CAD build for the part. Positions are in the model's coordinates, mm. A direction names the side the tool comes from. Give positions to 0.01 mm unless a question says otherwise; leave off trailing zeros. Loops run counter-clockwise (first coordinate to the right, second up) from the corner with the lowest first, then second, coordinate; pieces in that order, holes last.
```python
from build123d import *

# Parameters (mm, degrees)
M3_THREAD_ENVELOPE_SELECT_HARDWARE_START = 40
SKETCH1_R                                = 1.5
M3_THREAD_ENVELOPE_SELECT_HARDWARE_DEPTH = 7.5
THUMB_HEAD_START                         = 47.5
SKETCH2_R                                = 4
THUMB_HEAD_DEPTH                         = 4
DRIVER_SLOT_START                        = 50
SKETCH3_W                                = 1.2
SKETCH3_H                                = 10
DRIVER_SLOT_DEPTH                        = 3


with BuildPart() as part:
    # Sketch1 → M3_thread_envelope_select_hardware (new body)
    with BuildSketch(Plane.XY.offset(M3_THREAD_ENVELOPE_SELECT_HARDWARE_START)):
        with Locations((-20, 0)):
            Circle(SKETCH1_R)
    extrude(amount=M3_THREAD_ENVELOPE_SELECT_HARDWARE_DEPTH)

    # Sketch2 → Thumb_head (add)
    with BuildSketch(Plane.XY.offset(THUMB_HEAD_START)):
        with Locations((-20, 0)):
            Circle(SKETCH2_R)
    extrude(amount=THUMB_HEAD_DEPTH)

    # Sketch3 → Driver_slot (cut)
    with BuildSketch(Plane.XY.offset(DRIVER_SLOT_START)):
        with Locations((-20, 0)):
            Rectangle(SKETCH3_W, SKETCH3_H)
    extrude(amount=DRIVER_SLOT_DEPTH, mode=Mode.SUBTRACT)


solid = part.part
```
1. Probe line 1 along Z through (x, y) = (-19.5, 3.25); line 2 along Z through (x, y) = (-22.75, -0.25); line 3 along Y through (x, z) = (-20, 44.5). List the from-to ranges inside material, lowest first.
Responses:
line 1: z = 47.5 to 50
line 2: z = 47.5 to 51.5
line 3: y = -1.5 to 1.5
2. Saw through at D-D, the plane z = 49. List the corners of the cut face in (x, y), and give its area (3 significant figures).
Responses:
outline: circle Ø8 at (-20, 0)
area: 50.3 mm2
3. Pull direction X, two halves, no side cores. Call faces 4 (the face through (-20.6, 0, 51)), 5 (the face through (-22, 0, 51.5)), 6 (the face through (-20.867, -3.905, 49.472)): released by +X, released by -X, zero draft, split by the parting line, or undercut.
Responses:
face 4: undercut
face 5: zero draft
face 6: split by the parting line
4. Saw through at C-C, the plane z = 50.25. List the corners of the cut face in (x, y).
Responses:
outline: (-20.6, -3.95) - (-20.6, 3.95) arc R4 ccw to start; (-19.4, -3.95) arc R4 ccw to (-19.4, 3.95) - close
5. Drop flat-ended pins along their axis: pin 1 (1 mm diameter, centred on x = -23, z = 42, fed in from -Y); pin 2 (1.5 mm diameter, centred on x = -20.5, z = 42.5, fed in from +Y); pin 3 (3 mm diameter, centred on y = -3, z = 48.5, fed in from +X); pin 4 (2.5 mm diameter, centred on x = -19.5, y = -2, fed in from -Z). Give the stop position or say it passes through.
Responses:
pin 1: passes through
pin 2: stops at y = 1.5
pin 3: stops at x = -16.29
pin 4: stops at z = 40
6. Tool access for faces 1 (the face through (-19.4, 0, 51)), 2 (the face through (-20, 0, 40)), 3 (the face through (-21.5, 0.07, 43.7)): list every direction of +Z, -Z, +X, -X, +Y, -Y with a clear straight run to the whole face (end or side of a thin tool).
Responses:
face 1: +Z, +Y, -Y
face 2: -Z, +X, -X, +Y, -Y
face 3: -Z
7. Saw through at A-A, the plane y = 0. List the corners of the cut face in (x, z).
Responses:
outline: (-24, 47.5) - (-21.5, 47.5) - (-21.5, 40) - (-18.5, 40) - (-18.5, 47.5) - (-16, 47.5) - (-16, 51.5) - (-19.4, 51.5) - (-19.4, 50) - (-20.6, 50) - (-20.6, 51.5) - (-24, 51.5) - close
8. Saw through at B-B, the plane x = -20. List the corners of the cut face in (y, z), and give its area (3 significant figures).
Responses:
outline: (-4, 47.5) - (-1.5, 47.5) - (-1.5, 40) - (1.5, 40) - (1.5, 47.5) - (4, 47.5) - (4, 50) - (-4, 50) - close
area: 42.5 mm2
